Work out the finished part from the listing and answer in its coordinate system (mm). A direction names the side the tool comes from. Give positions to 0.01 mm unless a question says otherwise; leave off trailing zeros. Order: outer loops, then holes, each group sorted by start corner. A loop starts at its lowest first (then second) coordinate and runs counter-clockwise, first axis right, second up.
```python
from build123d import *

# Parameters (mm, degrees)
CYLINDER077_R          = 3
CYLINDER077_DEPTH      = 32
CYLINDER077_ROLL_ANGLE = -90
CYLINDER076_R          = 3
CYLINDER076_DEPTH      = 32
CYLINDER076_ROLL_ANGLE = -90
PRISM002_DEPTH         = 10
PRISM002_ROLL_ANGLE    = -90
PRISM003_DEPTH         = 10
PRISM003_ROLL_ANGLE    = -90
CYLINDER071_R          = 1.75
CYLINDER071_DEPTH      = 32
CYLINDER071_ROLL_ANGLE = -90
CYLINDER072_R          = 1.75
CYLINDER072_DEPTH      = 32
CYLINDER072_ROLL_ANGLE = -90
BOX055_W               = 20
BOX055_H               = 16
BOX055_DEPTH           = 56
PAD009_DEPTH           = 25
CHAMFER109_SIZE        = 5


with BuildPart() as cilindro018:
    # Cylinder077 → Cylinder077 (new body)
    with BuildSketch(Plane.XY):
        Circle(CYLINDER077_R)
    extrude(amount=CYLINDER077_DEPTH)


with BuildPart() as cilindro018_1:
    # Cylinder077 roll: moved
    add(cilindro018.part.rotate(Axis((0, 0, 0), (1, 0, 0)), CYLINDER077_ROLL_ANGLE))


with BuildPart() as cilindro018_2:
    # Cylinder077 placement: moved
    add(cilindro018_1.part.moved(Location((8, 116, 84))))


with BuildPart() as fusion059:
    # Cylinder076 → Cylinder076 (new body)
    with BuildSketch(Plane.XY):
        Circle(CYLINDER076_R)
    extrude(amount=CYLINDER076_DEPTH)


with BuildPart() as fusion059_1:
    # Cylinder076 roll: moved
    add(fusion059.part.rotate(Axis((0, 0, 0), (1, 0, 0)), CYLINDER076_ROLL_ANGLE))


with BuildPart() as fusion059_2:
    # Cylinder076 placement: moved
    add(fusion059_1.part.moved(Location((18, 116, 84))))

    # Fusion059: union Cilindro018
    add(cilindro018_2.part)


with BuildPart() as prisma001:
    # Prism002 → Prism002 (new body)
    with BuildSketch(Plane.XY):
        Polygon((3.3, 0), (1.65, 2.857884), (-1.65, 2.857884), (-3.3, 0), (-1.65, -2.857884), (1.65, -2.857884), align=None)
    extrude(amount=PRISM002_DEPTH)


with BuildPart() as prisma001_1:
    # Prism002 roll: moved
    add(prisma001.part.rotate(Axis((0, 0, 0), (1, 0, 0)), PRISM002_ROLL_ANGLE))


with BuildPart() as prisma001_2:
    # Prism002 placement: moved
    add(prisma001_1.part.moved(Location((18, 85, 84))))


with BuildPart() as fusion058:
    # Prism003 → Prism003 (new body)
    with BuildSketch(Plane.XY):
        Polygon((3.3, 0), (1.65, 2.857884), (-1.65, 2.857884), (-3.3, 0), (-1.65, -2.857884), (1.65, -2.857884), align=None)
    extrude(amount=PRISM003_DEPTH)


with BuildPart() as fusion058_1:
    # Prism003 roll: moved
    add(fusion058.part.rotate(Axis((0, 0, 0), (1, 0, 0)), PRISM003_ROLL_ANGLE))


with BuildPart() as fusion058_2:
    # Prism003 placement: moved
    add(fusion058_1.part.moved(Location((8, 85, 84))))

    # Fusion058: union Prisma001
    add(prisma001_2.part)


with BuildPart() as cilindro012:
    # Cylinder071 → Cylinder071 (new body)
    with BuildSketch(Plane.XY):
        Circle(CYLINDER071_R)
    extrude(amount=CYLINDER071_DEPTH)


with BuildPart() as cilindro012_1:
    # Cylinder071 roll: moved
    add(cilindro012.part.rotate(Axis((0, 0, 0), (1, 0, 0)), CYLINDER071_ROLL_ANGLE))


with BuildPart() as cilindro012_2:
    # Cylinder071 placement: moved
    add(cilindro012_1.part.moved(Location((8, 90, 84))))


with BuildPart() as fusion055:
    # Cylinder072 → Cylinder072 (new body)
    with BuildSketch(Plane.XY):
        Circle(CYLINDER072_R)
    extrude(amount=CYLINDER072_DEPTH)


with BuildPart() as fusion055_1:
    # Cylinder072 roll: moved
    add(fusion055.part.rotate(Axis((0, 0, 0), (1, 0, 0)), CYLINDER072_ROLL_ANGLE))


with BuildPart() as fusion055_2:
    # Cylinder072 placement: moved
    add(fusion055_1.part.moved(Location((18, 90, 84))))

    # Fusion055: union Cilindro012
    add(cilindro012_2.part)


with BuildPart() as cubo005:
    # Box055 → Box055 (new body)
    with BuildSketch(Plane(origin=(3.5, 97.5, 79.5), x_dir=(1, 0, 0), z_dir=(0, 0, 1))):
        with Locations((10, 8)):
            Rectangle(BOX055_W, BOX055_H)
    extrude(amount=BOX055_DEPTH)


with BuildPart() as obj1:
    # Sketch014 → Pad009 (new body)
    with BuildSketch(Plane(origin=(0, 93, 0), x_dir=(-1, 0, 0), z_dir=(0, 1, 0))):
        Polygon((-43.087208, 41.265208), (-29.956285, 89.24578), (16.5937, 98.48838), (-20.850395, 33.106079), (-48.138032, 40.573932), (-47.610101, 42.502996), align=None)
    extrude(amount=PAD009_DEPTH)

    # Cut096: cut Cubo005
    add(cubo005.part, mode=Mode.SUBTRACT)

    # Cut097: cut Fusion055
    add(fusion055_2.part, mode=Mode.SUBTRACT)

    # Cut101: cut Fusion058
    add(fusion058_2.part, mode=Mode.SUBTRACT)

    # Cut102: cut Fusion059
    add(fusion059_2.part, mode=Mode.SUBTRACT)

    # Chamfer109
    chamfer109_edges = [obj1.edges().sort_by_distance(p)[0] for p in [
        (-16.5937, 105.5, 98.48838),
    ]]
    chamfer(chamfer109_edges, length=CHAMFER109_SIZE)


solid = obj1.part
```
1. Which of the six approach directions +Z, -Z, +X, -X, +Y, -Y give full straight-line access (tool end or side, diameter ignored) to faces 4 (the face through (45.4, 105.3, 41.9)), 5 (the face through (23.5, 105, 85)), 6 (the face through (5.537, 93.986, 82.551))?
Findings below:
face 4: +Z, +Y, -Y
face 5: +Z
face 6: -Y
2. Given P1, Ø1, axis at x = 18.5, y = 94, coming from the -Z side; P2, Ø10, axis at y = 104, z = 75.5, coming from the +X side; P3, Ø3, axis at x = 19, z = 83.5, coming from the +Y side; P4, Ø3, axis at x = 8, z = 84, coming from the -Y side, each flat-ended and moving along its own axis, determine where each tip first touches the part or whether it passes through.
Findings below:
P1: stops at z = 36.34
P2: stops at x = 35.09
P3: stops at y = 116
P4: passes through
3. The part is cut by section A-A (x = 18). Write down the section's boundary in (y, z), then the cut area to 3 significant figures.
Findings below:
outline: (93, 38.08) - (118, 38.08) - (118, 81) - (116, 81) - (116, 82.25) - (113.5, 82.25) - (113.5, 79.5) - (97.5, 79.5) - (97.5, 82.25) - (95, 82.25) - (95, 81.14) - (93, 81.14) - close; (93, 86.86) - (95, 86.86) - (95, 85.75) - (97.5, 85.75) - (97.5, 91.62) - (93, 91.62) - close; (113.5, 85.75) - (116, 85.75) - (116, 87) - (118, 87) - (118, 91.62) - (113.5, 91.62) - close
area: 1,100 mm2
4. The part is cut by section B-B (y = 104.25). Write down the section's boundary in (x, z).
Findings below:
outline: (-14.11, 94.15) - (20.85, 33.11) - (48.14, 40.57) - (47.61, 42.5) - (43.09, 41.27) - (29.96, 89.25) - (23.5, 90.53) - (23.5, 79.5) - (3.5, 79.5) - (3.5, 94.5) - (-11.69, 97.51) - close
5. The part is cut by section D-D (z = 77.5). Write down the section's boundary in (x, y), then the cut area to 3 significant figures.
Findings below:
outline: (-4.57, 93) - (33.17, 93) - (33.17, 118) - (-4.57, 118) - close
area: 944 mm2
6. The mould has two halves that part along X. Classify faces 1 (the face through (17, 93, 66)), 2 (the face through (8, 94, 86.858)), 3 (the face through (47.88, 105.32, 41.52)): pulls with the +X half, pulls with the -X half, needs draft (parallel to the pull), parting line crosses it, or undercut.
Findings below:
face 1: needs draft
face 2: undercut
face 3: pulls with the +X half
7. Straight lines are drawn through the part: probe 1 along X at (y, z) = (95.55, 84); probe 2 along X at (y, z) = (112.5, 80); probe 3 along Z at (x, y) = (8, 115.55). For each, find the intervals that lie inside material, in ascending order.
Findings below:
probe 1: x = -8.3 to 6.25, 9.75 to 16.25, 19.75 to 31.39
probe 2: x = -6.01 to 3.5, 23.5 to 32.49
probe 3: z = 55.54 to 82.25, 85.75 to 93.61
8. The part is cut by section C-C (x = 8). Write down the section's boundary in (y, z), then the cut area to 3 significant figures.
Findings below:
outline: (93, 55.54) - (118, 55.54) - (118, 81) - (116, 81) - (116, 82.25) - (113.5, 82.25) - (113.5, 79.5) - (97.5, 79.5) - (97.5, 82.25) - (95, 82.25) - (95, 81.14) - (93, 81.14) - close; (93, 86.86) - (95, 86.86) - (95, 85.75) - (97.5, 85.75) - (97.5, 93.61) - (93, 93.61) - close; (113.5, 85.75) - (116, 85.75) - (116, 87) - (118, 87) - (118, 93.61) - (113.5, 93.61) - close
area: 685 mm2
